CAD build for the part. Positions are in the model's coordinates, mm. Face numbers are marked on the shaded views. A direction names the side the tool comes from. Coordinates: 2 decimals unless noted, no trailing zeros. Order: outer loops, then holes, each group sorted by start corner. A loop starts at its lowest first (then second) coordinate and runs counter-clockwise, first axis right, second up. Notation, with made-up numbers: (-40, -17) - (8, -17) arc R27 ccw to (8, 20) - close; hole circle Ø8 at (-16.5, 26.25). An arc over 180 degrees is marked (long way). Write each question's results on one line, items separated by ' | '. Start each with the question number.
Q1. Pull direction Y, two halves, no side cores. Call the marked faces 1, 2 and 3: released by +Y, released by -Y, zero draft, split by the parting line, or undercut.
Q2. Which spindle directions (+Z, -Z, +X, -X, +Y, -Y) get a long thin tool onto all of the face, cutting with end or side? Do the marked faces 4, 5, 6 and 7. Say none if no direction does.
Q3. Band-saw the part on C-C, the plane y = 5.5. Write the cut outline in (x, z), then the cut area to 3 significant figures.
Q4. Wall check: probe 1 along Z at (x, y) = (-3, 7); probe 2 along Y at (x, z) = (-6.75, 3.5); probe 3 along X at (y, z) = (1.75, -3). Give the ranges that are in metal, low to high.
Q5. Band-saw the part on D-D, the plane y = 8.5. Write the cut outline in (x, z).
Q6. Pin check, flat tips, straight feed: P1, Ø2, axis at x = 3.5, y = 7, coming from the -Z side; P2, Ø5.5, axis at x = -4, y = 4, coming from the +Z side; P3, Ø0.9, axis at x = -9, y = 6, coming from the -Z side. Stop position of each tip, or through.
Q7. Band-saw the part on B-B, the plane z = 1.5. Write the cut outline in (x, y), then the cut area to 3 significant figures.
Q8. Band-saw the part on A-A, the plane x = 5.5. Write the cut outline in (y, z), then the cut area to 3 significant figures.
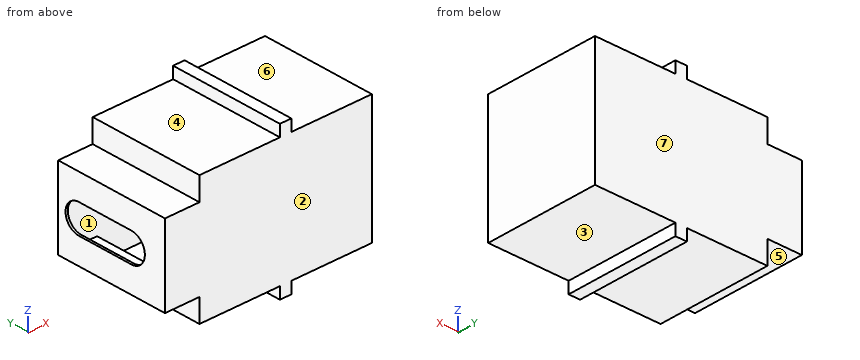
```python
from build123d import *

# Parameters (mm, degrees)
BOSS_EXTRUDE1_DEPTH = 10
SKETCH6_W           = 14.6
SKETCH6_H           = 10.6
SKETCH6_W_2         = 3
SKETCH6_H_2         = 6.6
BOSS_EXTRUDE4_DEPTH = 0.2
SKETCH7_W           = 14.6
SKETCH7_H           = 10.6
SKETCH7_W_2         = 3
SKETCH7_H_2         = 6.6
BOSS_EXTRUDE5_DEPTH = 0.2
CUT_EXTRUDE3_DEPTH  = 0.5


with BuildPart() as part:
    # Sketch1 → Boss-Extrude1 (new body)
    with BuildSketch(Plane(origin=(0, 0, 0), x_dir=(1, 0, 0), z_dir=(0, 1, 0))):
        Polygon((-10.028718685, -3.5), (-10.028718685, 3.5), (-7.028718685, 3.5), (-7.028718685, 5.5), (-0.028718685, 5.5), (-0.028718685, 6.5), (0.971281315, 6.5), (0.971281315, 5.5), (7.971281315, 5.5), (7.971281315, -5.5), (0.971281315, -5.5), (0.971281315, -6.5), (-0.028718685, -6.5), (-0.028718685, -5.5), (-7.028718685, -5.5), (-7.028718685, -3.5), align=None)
        Polygon((-9.828718685, 3.3), (-6.828718685, 3.3), (-6.828718685, 5.3), (0.171281315, 5.3), (0.771281315, 5.3), (7.771281315, 5.3), (7.771281315, -5.3), (0.771281315, -5.3), (0.171281315, -5.3), (-6.828718685, -5.3), (-6.828718685, -3.3), (-9.828718685, -3.3), align=None, mode=Mode.SUBTRACT)
    extrude(amount=BOSS_EXTRUDE1_DEPTH)

    # Sketch6 → Boss-Extrude4 (add)
    with BuildSketch(Plane(origin=(0, 0, 0), x_dir=(-1, 0, 0), z_dir=(0, -1, 0))):
        with Locations((-0.471281315, 0)):
            Rectangle(SKETCH6_W, SKETCH6_H)
        with Locations((8.328718685, 0)):
            Rectangle(SKETCH6_W_2, SKETCH6_H_2)
    extrude(amount=-BOSS_EXTRUDE4_DEPTH)

    # Sketch7 → Boss-Extrude5 (add)
    with BuildSketch(Plane(origin=(0, 10, 0), x_dir=(1, 0, 0), z_dir=(0, 1, 0))):
        with Locations((0.471281315, 0)):
            Rectangle(SKETCH7_W, SKETCH7_H)
        with Locations((-8.328718685, 0)):
            Rectangle(SKETCH7_W_2, SKETCH7_H_2)
    extrude(amount=-BOSS_EXTRUDE5_DEPTH)

    # Sketch8 → Cut-Extrude3 (cut)
    with BuildSketch(Plane.ZY.offset(10.028718685)):
        with BuildLine():
            Line((0, 9.314071319), (0, 5))
            Line((0, 5), (1.25, 5))
            Line((1.25, 5), (1.25, 8.064071319))
            ThreePointArc((1.25, 8.064071319), (0.883883476, 8.947954796), (0, 9.314071319))
        make_face()
        with BuildLine():
            Line((-1.25, 5), (0, 5))
            Line((0, 5), (0, 9.314071319))
            ThreePointArc((0, 9.314071319), (-0.883883476, 8.947954796), (-1.25, 8.064071319))
            Line((-1.25, 8.064071319), (-1.25, 5))
        make_face()
        with BuildLine():
            ThreePointArc((-1.25, 3.135928681), (-0.883883476, 2.252045204), (0, 1.885928681))
            Line((0, 1.885928681), (0, 5))
            Line((0, 5), (-1.25, 5))
            Line((-1.25, 5), (-1.25, 3.135928681))
        make_face()
        with BuildLine():
            Line((0, 5), (0, 1.885928681))
            ThreePointArc((0, 1.885928681), (0.883883476, 2.252045204), (1.25, 3.135928681))
            Line((1.25, 3.135928681), (1.25, 5))
            Line((1.25, 5), (0, 5))
        make_face()
    extrude(amount=-CUT_EXTRUDE3_DEPTH, mode=Mode.SUBTRACT)


solid = part.part
```
Results below:
1) face 1: undercut | face 2: released by -Y | face 3: zero draft
2) face 4: +Z, -X, +Y, -Y | face 5: -Z, -X, +Y, -Y | face 6: +Z, +X, +Y, -Y | face 7: +Z, -Z, +X, -X, +Y
3) outline: (-10.03, -3.5) - (-7.03, -3.5) - (-7.03, -5.5) - (-0.03, -5.5) - (-0.03, -6.5) - (0.97, -6.5) - (0.97, -5.5) - (7.97, -5.5) - (7.97, 5.5) - (0.97, 5.5) - (0.97, 6.5) - (-0.03, 6.5) - (-0.03, 5.5) - (-7.03, 5.5) - (-7.03, 3.5) - (-10.03, 3.5) - (-10.03, 1.25) - (-9.83, 1.25) - (-9.83, 3.3) - (-6.83, 3.3) - (-6.83, 5.3) - (7.77, 5.3) - (7.77, -5.3) - (-6.83, -5.3) - (-6.83, -3.3) - (-9.83, -3.3) - (-9.83, -1.25) - (-10.03, -1.25) - close | area: 12.9 mm²
4) probe 1: z = -5.5 to -5.3, 5.3 to 5.5 | probe 2: y = 0 to 0.2, 9.8 to 10 | probe 3: x = -10.03 to -9.83, 7.77 to 7.97
5) outline: (-10.03, -3.5) - (-7.03, -3.5) - (-7.03, -5.5) - (-0.03, -5.5) - (-0.03, -6.5) - (0.97, -6.5) - (0.97, -5.5) - (7.97, -5.5) - (7.97, 5.5) - (0.97, 5.5) - (0.97, 6.5) - (-0.03, 6.5) - (-0.03, 5.5) - (-7.03, 5.5) - (-7.03, 3.5) - (-10.03, 3.5) - (-10.03, 1.17) - (-9.83, 1.17) - (-9.83, 3.3) - (-6.83, 3.3) - (-6.83, 5.3) - (7.77, 5.3) - (7.77, -5.3) - (-6.83, -5.3) - (-6.83, -3.3) - (-9.83, -3.3) - (-9.83, -1.17) - (-10.03, -1.17) - close
6) P1: stops at z = -5.5 | P2: stops at z = 5.5 | P3: stops at z = -3.5
7) outline: (-10.03, 0) - (7.97, 0) - (7.97, 10) - (-10.03, 10) - close; hole (-9.83, 0.2) - (7.77, 0.2) - (7.77, 9.8) - (-9.83, 9.8) - close | area: 11.0 mm²
8) outline: (0, -5.5) - (10, -5.5) - (10, 5.5) - (0, 5.5) - close; hole (0.2, -5.3) - (9.8, -5.3) - (9.8, 5.3) - (0.2, 5.3) - close | area: 8.24 mm²
